Here's how the part is built. I have some questions about the finished solid (model axes, mm). Face numbers are marked on the shaded views. A direction names the side the tool comes from. Round coordinates to 2 decimals unless told otherwise and drop trailing zeros. Loops run counter-clockwise (first coordinate to the right, second up) from the corner with the lowest first, then second, coordinate; pieces in that order, holes last. Notation, with made-up numbers: M -20,49.25 L 3,49.25 A33 cw 3,84.25 Z; hole C 1.25,55 d4. An arc over 180 degrees is marked long. Put each result on its own line as item: value. Start each with the question number.
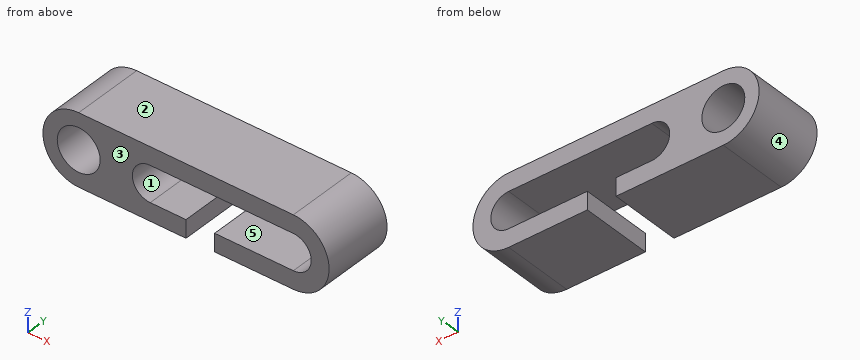
```python
from build123d import *

# Parameters (mm, degrees)
SKETCH1_R           = 3
BOSS_EXTRUDE1_DEPTH = 10


with BuildPart() as part:
    # Sketch1 → Boss-Extrude1 (new body)
    with BuildSketch(Plane(origin=(0, 0, 0), x_dir=(1, 0, 0), z_dir=(0, 1, 0))):
        with BuildLine():
            Line((-45.892533193, 15.021428325), (-30.892533193, 15.021428325))
            Line((-30.892533193, 15.021428325), (-30.892533193, 12.521428325))
            Line((-30.892533193, 12.521428325), (-35.892533193, 12.521428325))
            ThreePointArc((-35.892533193, 12.521428325), (-38.392533193, 10.021428325), (-35.892533193, 7.521428325))
            Line((-35.892533193, 7.521428325), (-15.892533193, 7.521428325))
            ThreePointArc((-15.892533193, 7.521428325), (-13.392533193, 10.021428325), (-15.892533193, 12.521428325))
            Line((-15.892533193, 12.521428325), (-26.892533193, 12.521428325))
            Line((-26.892533193, 12.521428325), (-26.892533193, 15.021428325))
            Line((-26.892533193, 15.021428325), (-15.892533193, 15.021428325))
            ThreePointArc((-15.892533193, 15.021428325), (-10.892533193, 10.021428325), (-15.892533193, 5.021428325))
            Line((-15.892533193, 5.021428325), (-45.892533193, 5.021428325))
            ThreePointArc((-45.892533193, 5.021428325), (-50.892533193, 10.021428325), (-45.892533193, 15.021428325))
        make_face()
        with Locations(Location((-45.892533193, 10.021428325, 0), (0, 0, 270))):
            Circle(SKETCH1_R, mode=Mode.SUBTRACT)
    extrude(amount=BOSS_EXTRUDE1_DEPTH)


solid = part.part
```
1) I'm going to push flat-ended pins straight in: P1, Ø1, axis at y = 5, z = -8.5, coming from the +X side; P2, Ø3, axis at y = 7, z = -11, coming from the +X side; P3, Ø2, axis at y = 3.5, z = -14.5, coming from the +X side; P4, Ø2, axis at y = 7, z = -13.5, coming from the -X side. Where does each tip first touch, or does it pass through?
2) Suppose I cut it at D-D (z = -14). Write out the boundary of the cut face in (x, y).
3) If I drill on probe 1 along X at (y, z) = (2.75, -10); probe 2 along Z at (x, y) = (-20, 3); probe 3 along X at (y, z) = (4, -9), over which ranges is the centre line in solid material (lowest first)? Write a range as from..to.
4) On a 3-axis mill with a long thin cutter (end or side, diameter ignored), from which of +Z, -Z, +X, -X, +Y, -Y can I reach the whole of each face in a straight line? I mean the marked faces 1 and 2. Say none if no direction works.
5) Suppose I cut it at B-B (y = 3.5). Write out the boundary of the cut face in (x, z), plus the area to 3 significant figures.
6) Suppose I cut it at C-C (z = -12). Write out the boundary of the cut face in (x, y), plus the area to 3 significant figures.
7) Suppose I cut it at A-A (x = -21). Write out the boundary of the cut face in (y, z).
8) If we mould it in two halves opening along Z, with no side actions, what happens to the marked faces 3, 4 and 5? For each: pulls with the +Z half, pulls with the -Z half, needs draft (parallel to the pull), parting line crosses it, or undercut.
Results are:
1. P1: x = -11
1. P2: x = -10.89
1. P3: x = -12.3
1. P4: x = -50.23
2. outline: M -48.92,0 L -30.89,0 L -30.89,10 L -48.92,10 Z; M -26.89,0 L -12.86,0 L -12.86,10 L -26.89,10 Z
3. probe 1: -50.89..-48.89, -42.89..-38.39, -13.39..-10.89
3. probe 2: -15.02..-12.52, -7.52..-5.02
3. probe 3: -50.79..-48.71, -43.07..-38.17, -13.61..-11
4. face 1: +Y, -Y
4. face 2: +Z, +X, -X, +Y, -Y
5. outline: M -45.89,-15.02 L -30.89,-15.02 L -30.89,-12.52 L -35.89,-12.52 A2.5 cw -35.89,-7.52 L -15.89,-7.52 A2.5 cw -15.89,-12.52 L -26.89,-12.52 L -26.89,-15.02 L -15.89,-15.02 A5 ccw -15.89,-5.02 L -45.89,-5.02 A5 ccw Z; hole C -45.89,-10.02 d6
5. area: 221 mm²
6. outline: M -50.48,0 L -48.15,0 L -48.15,10 L -50.48,10 Z; M -43.64,0 L -37.42,0 L -37.42,10 L -43.64,10 Z; M -14.36,0 L -11.3,0 L -11.3,10 L -14.36,10 Z
6. area: 116 mm²
7. outline: M 0,-15.02 L 10,-15.02 L 10,-12.52 L 0,-12.52 Z; M 0,-7.52 L 10,-7.52 L 10,-5.02 L 0,-5.02 Z
8. face 3: needs draft
8. face 4: parting line crosses it
8. face 5: undercut
